```python
from build123d import *

# Parameters (mm, degrees)
SKETCH1_W           = 139.7
SKETCH1_H           = 149.225
BOSS_EXTRUDE1_DEPTH = 85.725
SKETCH2_W           = 49.2125
SKETCH2_H           = 22.225
BOSS_EXTRUDE2_DEPTH = 6.35
SKETCH3_R           = 15.875
BOSS_EXTRUDE3_DEPTH = 6.35


with BuildPart() as part:
    # Sketch1 → Boss-Extrude1 (new body)
    with BuildSketch(Plane(origin=(0, 0, 0), x_dir=(1, 0, 0), z_dir=(0, 1, 0))):
        with Locations((69.85, 74.6125)):
            Rectangle(SKETCH1_W, SKETCH1_H)
    extrude(amount=BOSS_EXTRUDE1_DEPTH)

    # Sketch2 → Boss-Extrude2 (add)
    with BuildSketch(Plane.ZY):
        with Locations((-29.36875, 42.8625)):
            Rectangle(SKETCH2_W, SKETCH2_H)
    extrude(amount=BOSS_EXTRUDE2_DEPTH)

    # Sketch3 → Boss-Extrude3 (add)
    with BuildSketch(Plane(origin=(139.7, 0, 0), x_dir=(0, 0, -1), z_dir=(1, 0, 0))):
        with Locations(Location((15.875, 42.8625, 0), (0, 0, 180))):
            Circle(SKETCH3_R)
    extrude(amount=BOSS_EXTRUDE3_DEPTH)


solid = part.part
```
Input: part model. Units: mm. Frame: model coordinates. A direction names the side the tool comes from. Give positions to 0.01 mm unless a question says otherwise; leave off trailing zeros. Loops run counter-clockwise (first coordinate to the right, second up) from the corner with the lowest first, then second, coordinate; pieces in that order, holes last. Notation, with made-up numbers: (-24.75, 56) -> (-3.75, 56) arc R6 cw to (-3.75, 65) -> close; hole circle Ø3 at (61.5, -26). An arc over 180 degrees is marked (long way). Use a Markdown table: item, result.
Q1. Section query D-D, the plane y = 20. Return the cut outline in (x, z) (3 decimals), plus the area to 3 significant figures.
Entries:
| item | result |
|---|---|
| outline | (0, -149.225) -> (139.7, -149.225) -> (139.7, 0) -> (0, 0) -> close |
| area | 20,800 mm² |
Q2. Access query for faces 1 (the flat face through (-3, 43, -53.975)), 2 (the cylindrical face through (142.831, 38.094, -0.733)), 3 (the flat face through (-3, 53.975, -30)), 4 (the flat face through (-3, 43, -4.762)). Directions: +Z, -Z, +X, -X, +Y, -Y. A direction counts if a zero-diameter tool reaches every point of the face in a straight line with its end or side. Return the directions, or none.
Entries:
| item | result |
|---|---|
| face 1 | -Z, -X, +Y, -Y |
| face 2 | +X |
| face 3 | +Z, -Z, -X, +Y |
| face 4 | +Z, -X, +Y, -Y |
Q3. First-contact query: P1, Ø12, axis at y = 75.5, z = -89.5, coming from the +X side; P2, Ø3, axis at x = -2, z = -23.5, coming from the +Y side (3 decimals); P3, Ø1.9, axis at x = -3, y = 38, coming from the +Z side. Flat tips, straight axial feed; report the tip coordinate or a pass-through.
Entries:
| item | result |
|---|---|
| P1 | stops at x = 139.7 |
| P2 | stops at y = 53.975 |
| P3 | stops at z = -4.76 |
Q4. Section query C-C, the plane z = -104.5. Return the cut outline in (x, y) (3 decimals).
Entries:
| item | result |
|---|---|
| outline | (0, 0) -> (139.7, 0) -> (139.7, 85.725) -> (0, 85.725) -> close |
Q5. Ray query, probe 1 along X at (y, z) = (62.5, -141). Return the intervals inside material, ascending. Write a range as from..to.
Entries:
| item | result |
|---|---|
| probe 1 | x = 0..139.7 |
Q6. Section query A-A, the plane z = -52. Return the cut outline in (x, y) (3 decimals), plus the area to 3 significant figures.
Entries:
| item | result |
|---|---|
| outline | (-6.35, 31.75) -> (0, 31.75) -> (0, 0) -> (139.7, 0) -> (139.7, 85.725) -> (0, 85.725) -> (0, 53.975) -> (-6.35, 53.975) -> close |
| area | 12,100 mm² |
